from build123d import *

# Parameters (mm, degrees)
F1_DEPTH = 38.1
F2_SIZE  = 5.08
F3_SIZE  = 5.08
F4_SIZE  = 5.08
F5_T     = -3.81
F6_DEPTH = 25.4
F0_W     = 3.5
F0_H     = 2.25
F7_DEPTH = 38.1


with BuildPart() as f1:
    # F0 (on Top) → F1 (new body)
    with BuildSketch(Plane.XY):
        Polygon((52.1997908056, -19.3742188337), (48.6997908056, -19.3742188337), (40.4497908056, -19.3742188337), (50.4497908056, -57.4742188337), (60.4497908056, -57.4742188337), (60.4497908056, -19.3742188337), align=None)
    extrude(amount=-F1_DEPTH)

    # F2
    f2_edges = [f1.edges().sort_by_distance(p)[0] for p in [
        (50.449791, -57.474219, -19.05),
    ]]
    chamfer(f2_edges, length=F2_SIZE)

    # F3
    f3_edges = [f1.edges().sort_by_distance(p)[0] for p in [
        (49.160139, -52.560646, -19.05),
    ]]
    chamfer(f3_edges, length=F3_SIZE)

    # F4
    f4_edges = [f1.edges().sort_by_distance(p)[0] for p in [
        (47.870487, -47.647073, -19.05),
    ]]
    chamfer(f4_edges, length=F4_SIZE)

    # F5
    f5_openings = [f1.faces().sort_by_distance(p)[0] for p in [
        (52.764065, -35.551883, -38.1),
    ]]
    offset(amount=F5_T, openings=f5_openings)

    # F6 (cut): a face of the model
    f6_faces = [f1.faces().sort_by_distance(p)[0] for p in [
        (52.597107383, -34.5596646163, -3.81),
    ]]
    extrude(f6_faces, amount=-F6_DEPTH, mode=Mode.SUBTRACT)

    # F0 (on Top) → F7 (join)
    with BuildSketch(Plane.XY):
        with Locations((50.4497908056, -18.2492188337)):
            Rectangle(F0_W, F0_H)
        Polygon((45.4497908056, -17.1242188337), (48.6997908056, -17.1242188337), (52.1997908056, -17.1242188337), (54.9497908056, -17.1242188337), (54.9497908056, -15.8742188337), (45.4497908056, -15.8742188337), align=None)
        Polygon((48.6997908056, -13.3742188337), (45.4497908056, -15.8742188337), (54.9497908056, -15.8742188337), (52.1997908056, -13.3742188337), align=None)
    extrude(amount=-F7_DEPTH)


solid = f1.part
The model under review builds one solid part; all positions refer to its coordinate system, in mm. A direction names the side the tool comes from. Coordinates: 2 decimals unless noted, no trailing zeros. Write each loop counter-clockwise with the first axis right and the second up, starting at its lowest first coordinate (ties: lowest second). Pieces come first, ordered by that corner, then holes. Notation, with made-up numbers: (10, 88) - (62, 88) arc R34 cw to (62, 124) - close; hole circle Ø11 at (42, -29). An arc over 180 degrees is marked (long way). Answer as a JSON object with one key per item and string values. Group by question number.
1. Mouldability with a two-part tool opening along Y and no side actions: class faces 6 (the face through (52.2, -18, -19)), 7 (the face through (48, -35, -38.1)), 8 (the face through (53.59, -14.64, -18.78)), 9 (the face through (54.37, -56.58, -18.78)) as pulls with the +Y half, pulls with the -Y half, needs draft (parallel to the pull), parting line crosses it, or undercut.
2. To check wall thickness, follow probe 1 along Y at (x, z) = (54.75, -35); probe 2 along Y at (x, z) = (54.5, -23); probe 3 along Y at (x, z) = (59.25, -36.5). State the ranges of each line that lie inside material, in increasing order.
3. Add section B-B (y = -29). Give the boundary of the cut face in (x, z).
4. Add section D-D (x = 42.75). Give the boundary of the cut face in (y, z).
5. Add section A-A (z = -19). Give the boundary of the cut face in (x, y), plus the area to 3 significant figures.
6. Clearance check with flat-ended pins moving along their axes: pin 1 Ø4 at (x, z) = (55, -17) entering from +Y; pin 2 Ø6 at (y, z) = (-50.5, -13.5) entering from -X; pin 3 Ø9 at (y, z) = (-41.5, -15.5) entering from -X; pin 4 Ø10 at (x, y) = (48, -18.5) entering from +Z. State where each tip first meets the part, or that it passes through.
7. Add section C-C (x = 58.25). Give the boundary of the cut face in (y, z).
8. Machinability: for faces 1 (the face through (48.7, -18, -19)), 2 (the face through (54.95, -16.5, -18.8)), 3 (the face through (48, -35, 0)), 4 (the face through (51, -23.184, -19)), 5 (the face through (54, -17.124, -19)), which of the approach directions +Z, -Z, +X, -X, +Y, -Y give a long, thin tool a straight path to every point of the face, cutting with its end or side? Answer none if there is none.
Findings:
{
 "1": {"face 6": "undercut", "face 7": "needs draft", "face 8": "pulls with the +Y half", "face 9": "pulls with the -Y half"},
 "2": {"probe 1": "-56.87 to -51.13, -23.18 to -19.37, -17.12 to -15.69", "probe 2": "-56.68 to -50.75, -23.18 to -19.37, -17.12 to -15.47", "probe 3": "-57.47 to -19.37"},
 "3": {"outline": "(42.98, -38.1) - (46.92, -38.1) - (46.92, 0) - (42.98, 0) - close; (56.64, -38.1) - (60.45, -38.1) - (60.45, 0) - (56.64, 0) - close"},
 "4": {"outline": "(-28.14, -38.1) - (-19.37, -38.1) - (-19.37, 0) - (-28.14, 0) - close"},
 "5": {"outline": "(40.45, -19.37) - (46.58, -42.73) - (50.68, -51.88) - (53.18, -55.66) - (55.53, -57.47) - (60.45, -57.47) - (60.45, -19.37) - (52.2, -19.37) - (52.2, -17.12) - (54.95, -17.12) - (54.95, -15.87) - (52.2, -13.37) - (48.7, -13.37) - (45.45, -15.87) - (45.45, -17.12) - (48.7, -17.12) - (48.7, -19.37) - close; hole (45.39, -23.18) - (50.19, -41.46) - (54.03, -50.04) - (56.01, -53.03) - (56.64, -53.52) - (56.64, -23.18) - close", "area": "377 mm²"},
 "6": {"pin 1": "y = -14.1", "pin 2": "x = 48.71", "pin 3": "x = 45.08", "pin 4": "z = 0"},
 "7": {"outline": "(-57.47, -38.1) - (-19.37, -38.1) - (-19.37, 0) - (-57.47, 0) - close"},
 "8": {"face 1": "+Z, -Z, -X", "face 2": "+Z, -Z, +X, +Y", "face 3": "+Z, +X, -X, +Y, -Y", "face 4": "+Z, -Z", "face 5": "+Z, -Z, +X"}
}
